from build123d import *

# Parameters (mm, degrees)
SKETCH1_W           = 50
SKETCH1_H           = 18
BOSS_EXTRUDE1_DEPTH = 15
SKETCH2_W           = 7.9
SKETCH2_H           = 8.5
CUT_EXTRUDE1_DEPTH  = 15
SKETCH3_W           = 47
SKETCH3_H           = 15
CUT_EXTRUDE2_DEPTH  = 4
SKETCH4_W           = 6.9
SKETCH4_H           = 14
SKETCH4_R           = 1.5
BOSS_EXTRUDE2_DEPTH = 1
LPATTERN1_COUNT     = 5
LPATTERN1_PITCH     = 9.8
SKETCH5_W           = 6.9
SKETCH5_H           = 6.9
SKETCH5_R           = 1.5
BOSS_EXTRUDE3_DEPTH = 1
LPATTERN2_COUNT     = 5
LPATTERN2_PITCH     = 9.8


with BuildPart() as part:
    # Sketch1 → Boss-Extrude1 (new body)
    with BuildSketch(Plane(origin=(0, 0, 0), x_dir=(1, 0, 0), z_dir=(0, 1, 0))):
        Rectangle(SKETCH1_W, SKETCH1_H)
    extrude(amount=BOSS_EXTRUDE1_DEPTH)

    # Sketch2 → Cut-Extrude1 (cut)
    with BuildSketch(Plane.XY.offset(9)):
        with Locations((-19.75, 10.75)):
            Rectangle(SKETCH2_W, SKETCH2_H)
        with Locations((-10.05, 10.75)):
            Rectangle(SKETCH2_W, SKETCH2_H)
        with Locations((-0.35, 10.75)):
            Rectangle(SKETCH2_W, SKETCH2_H)
        with Locations((9.35, 10.75)):
            Rectangle(SKETCH2_W, SKETCH2_H)
        with Locations((19.05, 10.75)):
            Rectangle(SKETCH2_W, SKETCH2_H)
    extrude(amount=-CUT_EXTRUDE1_DEPTH, mode=Mode.SUBTRACT)

    # Sketch3 → Cut-Extrude2 (cut)
    with BuildSketch(Plane.XZ):
        Rectangle(SKETCH3_W, SKETCH3_H)
    extrude(amount=-CUT_EXTRUDE2_DEPTH, mode=Mode.SUBTRACT)

    # Sketch4 → Boss-Extrude2 (add)
    with BuildSketch(Plane(origin=(0, 6.5, 0), x_dir=(1, 0, 0), z_dir=(0, 1, 0))):
        with Locations((-19.75, -1.5)):
            Rectangle(SKETCH4_W, SKETCH4_H)
        with Locations(Location((-19.75, 2.05, 0), (0, 0, 180))):
            Circle(SKETCH4_R, mode=Mode.SUBTRACT)
    boss_extrude2 = extrude(amount=BOSS_EXTRUDE2_DEPTH)

    # LPattern1: Boss-Extrude2 ×5
    with Locations(*[(i * LPATTERN1_PITCH, 0, 0) for i in range(1, LPATTERN1_COUNT)]):
        add(boss_extrude2)

    # Sketch5 → Boss-Extrude3 (add)
    with BuildSketch(Plane(origin=(0, 7.5, 0), x_dir=(1, 0, 0), z_dir=(0, 1, 0))):
        with Locations((-19.75, 2.05)):
            Rectangle(SKETCH5_W, SKETCH5_H)
        with Locations(Location((-19.75, 2.05, 0), (0, 0, 180))):
            Circle(SKETCH5_R, mode=Mode.SUBTRACT)
    boss_extrude3 = extrude(amount=BOSS_EXTRUDE3_DEPTH)

    # LPattern2: Boss-Extrude3 ×5
    with Locations(*[(i * LPATTERN2_PITCH, 0, 0) for i in range(1, LPATTERN2_COUNT)]):
        add(boss_extrude3)


solid = part.part
Verification items for the finished model (mm, model axes). A direction names the side the tool comes from. Coordinates: 2 decimals unless noted, no trailing zeros. Order: outer loops, then holes, each group sorted by start corner. A loop starts at its lowest first (then second) coordinate and runs counter-clockwise, first axis right, second up. Notation, with made-up numbers: M -17.5,86 L 33.5,86 A19 ccw 33.5,98 Z; hole C 6.25,56.5 d6. An arc over 180 degrees is marked long. Return JSON: item names as keys, results as strings.
1) Thickness scan on L1, parallel to Z at x = -0.15, y = 7.6; L2, parallel to Z at x = -19.75, y = 7.05; L3, parallel to X at y = 9.5, z = 3.75. Record the ranges inside material, lowest first. Write a range as [from, to].
Answer list:
{"L1": "[-9, -6], [-5.5, -3.55], [-0.55, 1.4]", "L2": "[-9, -6], [-5.5, -3.55], [-0.55, 8.5]", "L3": "[-25, -23.7], [-15.8, -14], [-6.1, -4.3], [3.6, 5.4], [13.3, 15.1], [23, 25]"}
2) Access from +Z, -Z, +X, -X, +Y, -Y to the whole of each face (thin tool, end or side, straight path). Record for faces 1 (the flat face through (0, 4, 0)), 2 (the flat face through (10, 6.5, -2)), 3 (the flat face through (-10, 7.5, 5)).
Answer list:
{"face 1": "-Y", "face 2": "+Y", "face 3": "+Z, +Y"}
3) Release check for a two-part mould opening along X. For faces 4 (the flat face through (25, 7, 0)), 5 (the flat face through (-3.6, 7, 0)) record: +X half, -X half, draft (parallel to the pull), parting line (faces both ways), or undercut.
Answer list:
{"face 4": "+X half", "face 5": "undercut"}
4) Gauge pin test, flat ends, axial feed: pin 1 (10 mm diameter, centred on x = -11, z = -5, fed in from -Y); pin 2 (6 mm diameter, centred on x = -1, z = 2.5, fed in from +Y); pin 3 (4 mm diameter, centred on x = 9.65, z = -2.05, fed in from -Y); pin 4 (3.5 mm diameter, centred on x = -0.5, z = 3.5, fed in from +Y). Record the tip position at first contact, or that the pin passes through.
Answer list:
{"pin 1": "y = 0", "pin 2": "y = 8.5", "pin 3": "y = 4", "pin 4": "y = 7.5"}
5) Cross-section at B-B, the plane x = 19.45. Record the boundary of the cut face in (y, z).
Answer list:
{"outline": "M 0,-9 L 15,-9 L 15,-6 L 6.5,-6 L 6.5,-5.5 L 8.5,-5.5 L 8.5,-3.55 L 6.5,-3.55 L 6.5,-0.55 L 8.5,-0.55 L 8.5,1.4 L 7.5,1.4 L 7.5,8.5 L 6.5,8.5 L 6.5,9 L 0,9 L 0,7.5 L 4,7.5 L 4,-7.5 L 0,-7.5 Z"}
6) Cross-section at A-A, the plane y = 12.75. Record the boundary of the cut face in (x, z), and give its area (4 significant figures).
Answer list:
{"outline": "M -25,-9 L 25,-9 L 25,9 L 23,9 L 23,-6 L 15.1,-6 L 15.1,9 L 13.3,9 L 13.3,-6 L 5.4,-6 L 5.4,9 L 3.6,9 L 3.6,-6 L -4.3,-6 L -4.3,9 L -6.1,9 L -6.1,-6 L -14,-6 L -14,9 L -15.8,9 L -15.8,-6 L -23.7,-6 L -23.7,9 L -25,9 Z", "area": "307.5 mm2"}
